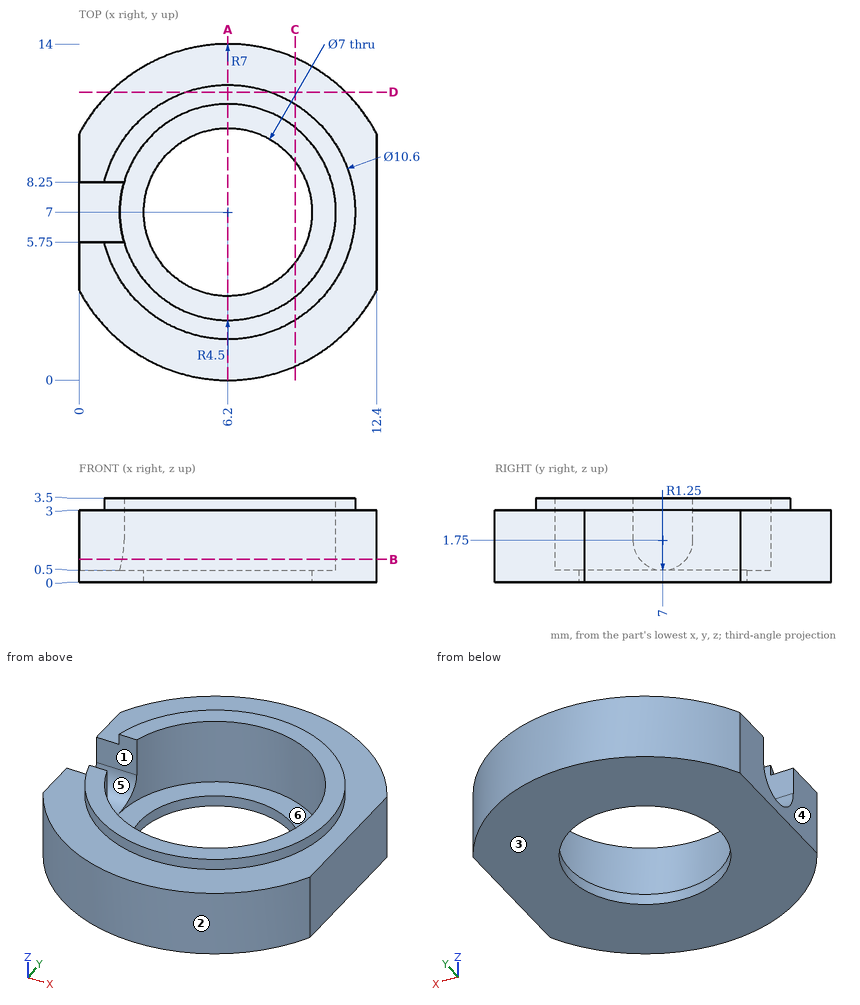
Drawing for the job (mm, zero at the part's lowest x, y, z). A direction names the side the tool comes from. Give positions to 0.01 mm unless a question says otherwise; leave off trailing zeros. Loops run counter-clockwise (first coordinate to the right, second up) from the corner with the lowest first, then second, coordinate; pieces in that order, holes last. Notation, with made-up numbers: M 7,58 L 46,58 A15 ccw 46,84 Z; hole C 6.5,41 d10. An arc over 180 degrees is marked long. One line per question, with ' | ' between items. Start each with the question number.
1. Saw through at B-B on z = 0.95. Give the cut face in (x, y).
2. Saw through at C-C on x = 9. Give the cut face in (y, z).
3. 3-axis set-ups, long thin cutter, end or side, ignore diameter. For the marked faces 4, 5 and 6: which of +Z, -Z, +X, -X, +Y, -Y reach the whole face in a straight line?
4. Flat gauge pins, fed straight in: pin 1 (0.9 mm diameter, centred on x = 1, z = 3, fed in from -Y); pin 2 (2 mm diameter, centred on x = 3.5, z = 1, fed in from -Y); pin 3 (1.5 mm diameter, centred on x = 4.5, z = 2.5, fed in from +Y). Where does each tip first touch, or does it go through?
5. Probe L1, parallel to Y at x = 6.2, z = 0.2; L2, parallel to Y at x = 6.5, z = 3.35; L3, parallel to X at y = 5.5, z = 1.7. List the from-to ranges inside material, lowest first. Write a range as from..to.
6. Saw through at D-D on y = 12. Give the cut face in (x, z), plus the area to 3 significant figures.
7. Two-plate mould, pull along Y, no slides. Class the marked faces 1, 2 and 3: pulls with the +Y half, pulls with the -Y half, needs draft (parallel to the pull), parting line crosses it, or undercut.
8. Saw through at A-A on x = 6.2. Give the cut face in (y, z).
Result sheet:
1) outline: M 0,3.75 A7 ccw 12.4,3.75 L 12.4,10.25 A7 ccw 0,10.25 L 0,7.96 L 1.8,7.96 A4.5 cw long 1.8,6.04 L 0,6.04 Z
2) outline: M 0.58,0 L 4.9,0 L 4.9,0.5 L 3.48,0.5 L 3.48,3.5 L 2.5,3.5 L 2.5,3 L 0.58,3 Z; M 9.1,0 L 13.42,0 L 13.42,3 L 11.5,3 L 11.5,3.5 L 10.52,3.5 L 10.52,0.5 L 9.1,0.5 Z
3) face 4: +Z, -Z, -X, +Y, -Y | face 5: +Z, -X | face 6: +Z
4) pin 1: stops at y = 1.86 | pin 2: stops at y = 0.21 | pin 3: stops at y = 13.94
5) L1: y = 0..3.5, 10.5..14 | L2: y = 1.71..2.51, 11.49..12.29 | L3: x = 0..1.96, 10.44..12.4
6) outline: M 1.3,0 L 11.1,0 L 11.1,3 L 7.96,3 L 7.96,3.5 L 4.44,3.5 L 4.44,3 L 1.3,3 Z | area: 31.2 mm^2
7) face 1: undercut | face 2: pulls with the -Y half | face 3: needs draft
8) outline: M 0,0 L 3.5,0 L 3.5,0.5 L 2.5,0.5 L 2.5,3.5 L 1.7,3.5 L 1.7,3 L 0,3 Z; M 10.5,0 L 14,0 L 14,3 L 12.3,3 L 12.3,3.5 L 11.5,3.5 L 11.5,0.5 L 10.5,0.5 Z
